Answer from the drawing. Dimensions are ordinates in mm from the lowest x, y and z of the part. A direction names the side the tool comes from. Give positions to 0.01 mm unless a question says otherwise; leave off trailing zeros. Order: outer loops, then holes, each group sorted by start corner. A loop starts at its lowest first (then second) coordinate and runs counter-clockwise, first axis right, second up. Notation, with made-up numbers: (89.5, 63) - (129.5, 63) arc R22 cw to (129.5, 86) - close; hole circle Ø9 at (43, 20.25). An arc over 180 degrees is marked (long way). Write each question's results on one line, items separated by ' | '.
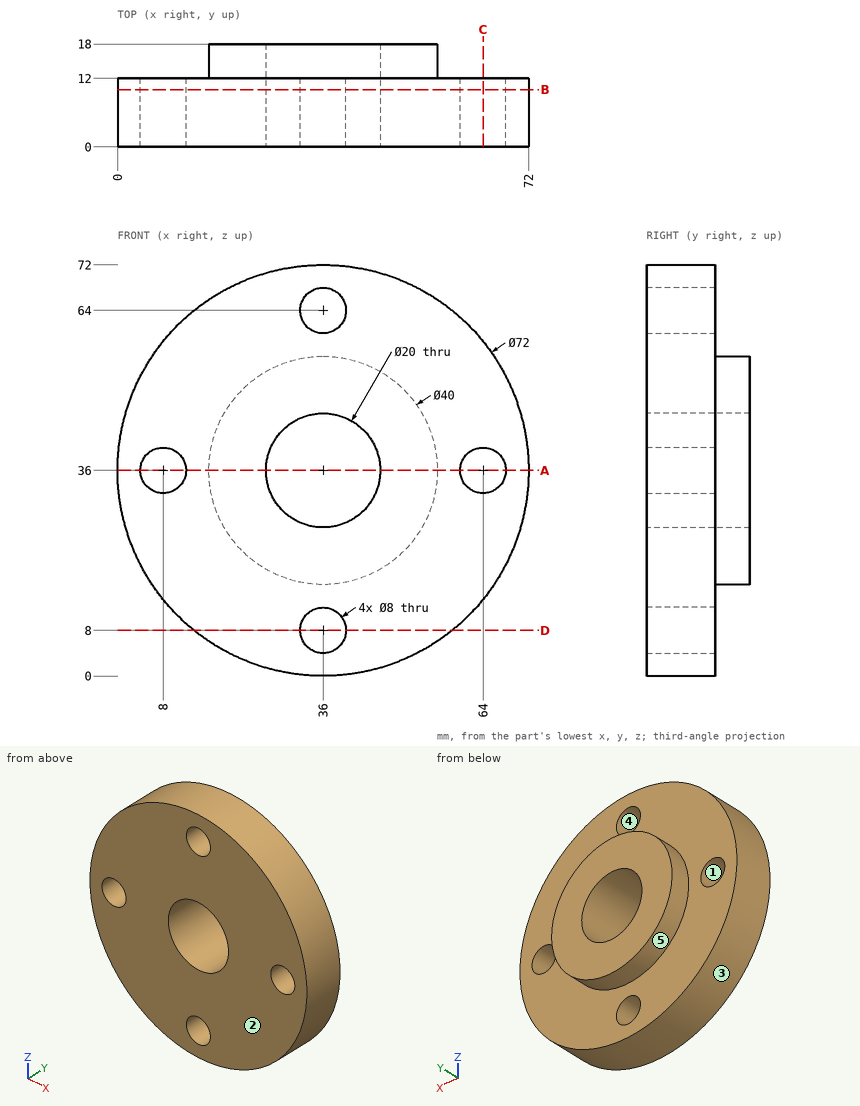
1. A cutting plane is placed at C-C, the plane x = 64. Write down the section's boundary in (y, z), then the cut area to 3 significant figures.
Answer list:
outline: (0, 13.37) - (12, 13.37) - (12, 32) - (0, 32) - close; (0, 40) - (12, 40) - (12, 58.63) - (0, 58.63) - close | area: 447 mm^2
2. A cutting plane is placed at A-A, the plane z = 36. Write down the section's boundary in (x, y), then the cut area to 3 significant figures.
Answer list:
outline: (0, 0) - (4, 0) - (4, 12) - (0, 12) - close; (12, 0) - (26, 0) - (26, 18) - (16, 18) - (16, 12) - (12, 12) - close; (46, 0) - (60, 0) - (60, 12) - (56, 12) - (56, 18) - (46, 18) - close; (68, 0) - (72, 0) - (72, 12) - (68, 12) - close | area: 552 mm^2
3. A cutting plane is placed at B-B, the plane y = 10. Write down the section's boundary in (x, z), then the cut area to 3 significant figures.
Answer list:
outline: circle Ø72 at (36, 36); hole circle Ø8 at (8, 36); hole circle Ø20 at (36, 36); hole circle Ø8 at (36, 8); hole circle Ø8 at (36, 64); hole circle Ø8 at (64, 36) | area: 3,560 mm^2
4. Straight lines are drawn through the part: line 1 (X direction, y = 3.75, z = 36); line 2 (Z direction, x = 39, y = 11.5); line 3 (Z direction, x = 61, y = 1.75). For each, find the intervals that lie inside material, in ascending order. Write a range as [from, to].
Answer list:
line 1: [0, 4], [12, 26], [46, 60], [68, 72] | line 2: [0.13, 5.35], [10.65, 26.46], [45.54, 61.35], [66.65, 71.87] | line 3: [10.1, 33.35], [38.65, 61.9]
5. Determine the mould class of the marked faces 1, 2 and 3 for opening direction X: +X half, -X half, draft (parallel to the pull), parting line (faces both ways), or undercut.
Answer list:
face 1: undercut | face 2: draft | face 3: parting line
6. A cutting plane is placed at D-D, the plane z = 8. Write down the section's boundary in (x, y), then the cut area to 3 significant figures.
Answer list:
outline: (13.37, 0) - (32, 0) - (32, 12) - (13.37, 12) - close; (40, 0) - (58.63, 0) - (58.63, 12) - (40, 12) - close | area: 447 mm^2
7. Given P1, Ø3, axis at y = 2.5, z = 7.5, coming from the +X side; P2, Ø5, axis at y = 5.5, z = 38, coming from the -X side; P3, Ø1.5, axis at x = 50.5, y = 12.5, coming from the +Z side, each flat-ended and moving along its own axis, determine where each tip first touches the part or whether it passes through.
Answer list:
P1: x = 59.81 | P2: x = 0 | P3: z = 69.19
8. A tool of negligible diameter and unlimited length cuts with its end or side. For the marked faces 4 and 5, from which of +Z, -Z, +X, -X, +Y, -Y can it reach the whole face along a straight path? Write none if from no direction.
Answer list:
face 4: +Y, -Y | face 5: +Y
